Part model, mm, in its own coordinate system. Face numbers are marked on the shaded views. A direction names the side the tool comes from. Give positions to 0.01 mm unless a question says otherwise; leave off trailing zeros. Order: outer loops, then holes, each group sorted by start corner. A loop starts at its lowest first (then second) coordinate and runs counter-clockwise, first axis right, second up. Notation, with made-up numbers: (83.5, 24.5) - (130.5, 24.5) arc R8 cw to (130.5, 36.5) - close; hole circle Ø10 at (40.5, -28.5). An arc over 180 degrees is marked (long way). One line per item, written item: value.
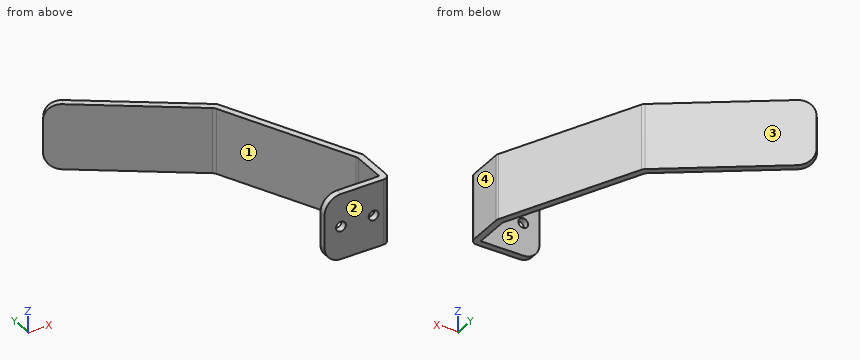
```python
from build123d import *

# Parameters (mm, degrees)
BOSS_EXTRUDE1_DEPTH = 10
FILLET1_R           = 2
FILLET2_R           = 5
SKETCH2_R           = 1.5
CUT_EXTRUDE1_DEPTH  = 3


with BuildPart() as part:
    # Sketch1 → Boss-Extrude1 (new, symmetric)
    with BuildSketch(Plane.XY):
        Polygon((0, 0), (20, 0), (20, 13), (0.982178222, 53.783850417), (-35.879663771, 79.594790052), (-37.026816644, 77.956485964), (-0.603956909, 52.452925014), (18, 12.556610675), (18, 2), (0, 2), align=None)
    extrude(amount=BOSS_EXTRUDE1_DEPTH, both=True)

    # Fillet1
    fillet1_edges = [part.edges().sort_by_distance(p)[0] for p in [
        (18, 12.556610675, 0),
        (-0.603956909, 52.452925014, 0),
        (0.982178222, 53.783850417, 0),
        (20, 13, 0),
        (20, 0, 0),
    ]]
    fillet(fillet1_edges, radius=FILLET1_R)

    # Fillet2
    fillet2_edges = [part.edges().sort_by_distance(p)[0] for p in [
        (-36.453240208, 78.775638008, -10),
        (0, 1, -10),
        (-36.453240208, 78.775638008, 10),
        (0, 1, 10),
    ]]
    fillet(fillet2_edges, radius=FILLET2_R)

    # Sketch2 → Cut-Extrude1 (cut)
    with BuildSketch(Plane.XZ):
        with Locations(Location((5, 0, 0), (0, 0, 270))):
            Circle(SKETCH2_R)
        with Locations(Location((15, 0, 0), (0, 0, 270))):
            Circle(SKETCH2_R)
    extrude(amount=-CUT_EXTRUDE1_DEPTH, mode=Mode.SUBTRACT)


solid = part.part
```
1) Pin check, flat tips, straight feed: pin 1 (1 mm diameter, centred on y = 34, z = 6.5, fed in from +X); pin 2 (6 mm diameter, centred on x = 3.5, z = 2.5, fed in from -Y); pin 3 (5 mm diameter, centred on x = -6, z = -1, fed in from +Y); pin 4 (10 mm diameter, centred on x = -5.5, z = 7, fed in from -Y). Stop position of each tip, or through.
Outcome:
pin 1: stops at x = 10.44
pin 2: stops at y = 0
pin 3: stops at y = 60.42
pin 4: stops at y = 52.19
2) Which spindle directions (+Z, -Z, +X, -X, +Y, -Y) get a long thin tool onto all of the face, cutting with end or side? Do the marked faces 1 and 2. Say none if no direction does.
Outcome:
face 1: +Z, -Z, -X
face 2: +Z, -Z, +X, -X, -Y
3) Cut at B-B, the plane x = 12. Give the cut face in (y, z), then the cut area to 3 significant figures.
Outcome:
outline: (0, -10) - (2, -10) - (2, 10) - (0, 10) - close; (25.42, -10) - (30.16, -10) - (30.16, 10) - (25.42, 10) - close
area: 135 mm^2
4) Drill centre lines: line 1 along X through (y, z) = (1.1, 0); line 2 along X through (y, z) = (0.45, 0); line 3 along Y through (x, z) = (4, -4). Where is each one in solid material? Low to high. Write a range as from..to.
Outcome:
line 1: x = 0..3.5, 6.5..13.5, 16.5..19.79
line 2: x = 0..3.5, 6.5..13.5, 16.5..19.26
line 3: y = 0..2, 42.58..47.31
5) Cut at A-A, the plane z = 0. Give the cut face in (x, y), then the cut area to 3 significant figures.
Outcome:
outline: (-37.03, 77.96) - (-1.04, 52.76) arc R2 cw to (-0.38, 51.97) - (17.81, 12.96) arc R2 cw to (18, 12.11) - (18, 2) - (16.5, 2) - (16.5, 0) - (18, 0) arc R2 ccw to (20, 2) - (20, 12.56) arc R2 ccw to (19.81, 13.4) - (1.21, 53.3) arc R2 ccw to (0.54, 54.09) - (-35.88, 79.59) - close; (0, 0) - (3.5, 0) - (3.5, 2) - (0, 2) - close; (6.5, 0) - (13.5, 0) - (13.5, 2) - (6.5, 2) - close
area: 227 mm^2
6) Mould opens along Y. For the marked faces 3, 4 and 5 say: released by +Y, released by -Y, zero draft, split by the parting line, or undercut.
Outcome:
face 3: released by +Y
face 4: zero draft
face 5: undercut
7) Cut at C-C, the plane z = 7.25. Give the cut face in (x, y).
Outcome:
outline: (-36.59, 77.65) - (-1.04, 52.76) arc R2 cw to (-0.38, 51.97) - (17.81, 12.96) arc R2 cw to (18, 12.11) - (18, 2) - (0.53, 2) - (0.53, 0) - (18, 0) arc R2 ccw to (20, 2) - (20, 12.56) arc R2 ccw to (19.81, 13.4) - (1.21, 53.3) arc R2 ccw to (0.54, 54.09) - (-35.44, 79.29) - close
8) Cut at D-D, the plane y = 10. Give the cut face in (x, z), then the cut area to 3 significant figures.
Outcome:
outline: (18, -10) - (20, -10) - (20, 10) - (18, 10) - close
area: 40.0 mm^2
